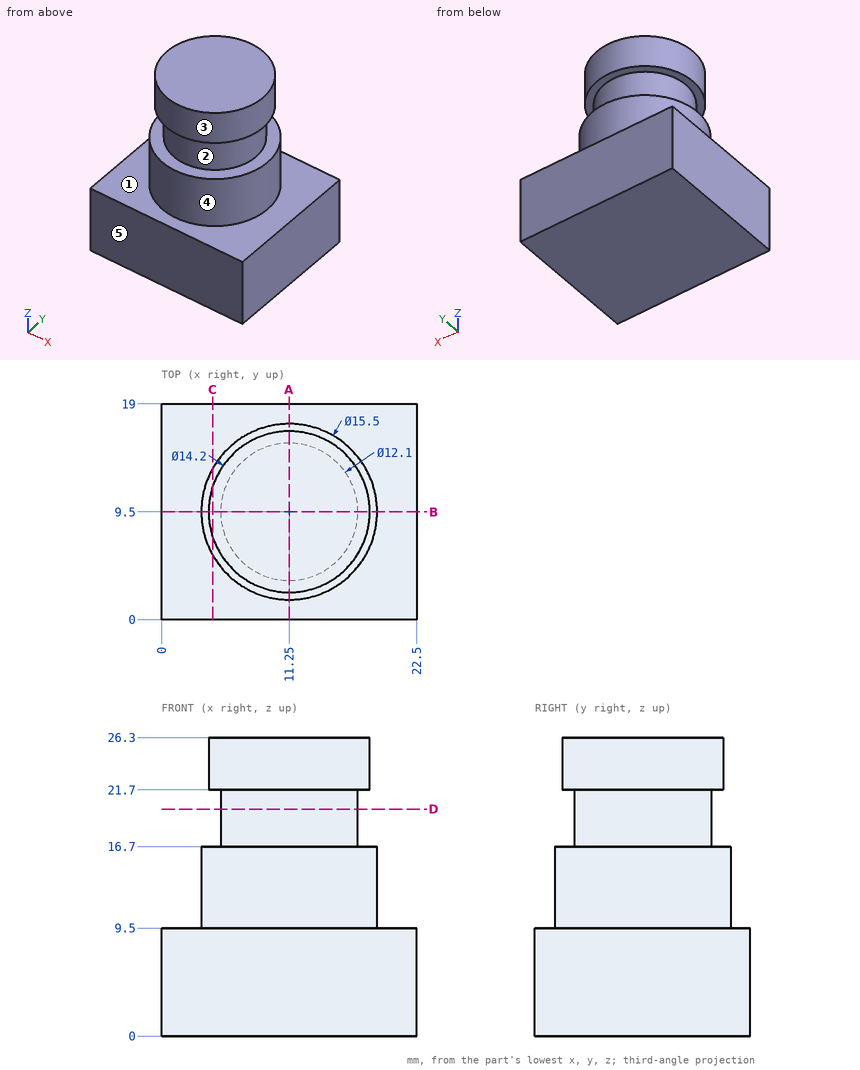
Design review of the part shown in the three views and the two pictorial views. Dimensions are in mm from the part's minimum x, y and z. A direction names the side the tool comes from. Round coordinates to 2 decimals unless told otherwise and drop trailing zeros. Loops run counter-clockwise (first coordinate to the right, second up) from the corner with the lowest first, then second, coordinate; pieces in that order, holes last. Notation, with made-up numbers: (89.5, 71) -> (116.5, 71) arc R18 cw to (116.5, 100) -> close; hole circle Ø2 at (-10.5, 89). An arc over 180 degrees is marked (long way). Return JSON: item names as keys, results as strings.
(1) For pin 1 (8 mm diameter, centred on y = 13, z = 3.5, fed in from -X); pin 2 (6 mm diameter, centred on y = 11, z = 22.5, fed in from +X); pin 3 (10 mm diameter, centred on y = 15.5, z = 22.5, fed in from -X), all flat-tipped, find the tip position at first contact; note any pin that passes through.
Solved:
{"pin 1": "x = 0", "pin 2": "x = 18.35", "pin 3": "x = 4.22"}
(2) Add section A-A on x = 11.25. Write out the cut boundary in (y, z), plus the area to 3 significant figures.
Solved:
{"outline": "(0, 0) -> (19, 0) -> (19, 9.5) -> (17.25, 9.5) -> (17.25, 16.7) -> (15.55, 16.7) -> (15.55, 21.7) -> (16.6, 21.7) -> (16.6, 26.3) -> (2.4, 26.3) -> (2.4, 21.7) -> (3.45, 21.7) -> (3.45, 16.7) -> (1.75, 16.7) -> (1.75, 9.5) -> (0, 9.5) -> close", "area": "418 mm2"}
(3) Add section C-C on x = 4.5. Write out the cut boundary in (y, z), plus the area to 3 significant figures.
Solved:
{"outline": "(0, 0) -> (19, 0) -> (19, 9.5) -> (13.31, 9.5) -> (13.31, 16.7) -> (5.69, 16.7) -> (5.69, 9.5) -> (0, 9.5) -> close; (7.3, 21.7) -> (11.7, 21.7) -> (11.7, 26.3) -> (7.3, 26.3) -> close", "area": "256 mm2"}
(4) Add section D-D on z = 20. Write out the cut boundary in (x, y), plus the area to 3 significant figures.
Solved:
{"outline": "circle Ø12.1 at (11.25, 9.5)", "area": "115 mm2"}
(5) For line 1 (Z direction, x = 19, y = 14.25); line 2 (Z direction, x = 16.75, y = 5.25); line 3 (X direction, y = 9.25, z = 14.5), list the stretches that pass through material, from the lowest coordinate up.
Solved:
{"line 1": "0 to 9.5", "line 2": "0 to 16.7, 21.7 to 26.3", "line 3": "3.5 to 19"}
(6) The part is to be moulded in two halves that separate along Z. For the marked faces 1, 2 and 3, say which applies: released by +Z, released by -Z, zero draft, split by the parting line, or undercut.
Solved:
{"face 1": "released by +Z", "face 2": "undercut", "face 3": "zero draft"}
(7) For the marked faces 4 and 5, list the 3-axis set-ups (+Z, -Z, +X, -X, +Y, -Y) from which the entire face can be reached by the end or side of a thin tool; tool diameter is ignored.
Solved:
{"face 4": "+Z", "face 5": "+Z, -Z, +X, -X, -Y"}
(8) Add section B-B on y = 9.5. Write out the cut boundary in (x, z).
Solved:
{"outline": "(0, 0) -> (22.5, 0) -> (22.5, 9.5) -> (19, 9.5) -> (19, 16.7) -> (17.3, 16.7) -> (17.3, 21.7) -> (18.35, 21.7) -> (18.35, 26.3) -> (4.15, 26.3) -> (4.15, 21.7) -> (5.2, 21.7) -> (5.2, 16.7) -> (3.5, 16.7) -> (3.5, 9.5) -> (0, 9.5) -> close"}
